```python
from build123d import *

# Parameters (mm, degrees)
F0_W     = 48
F0_H     = 1.6
F1_DEPTH = 48
F2_R     = 1.75
F2_R_2   = 1.8
F2_R_3   = 0.5
F3_DEPTH = 1.601
F4_W     = 48
F4_H     = 48
F4_R     = 1.75
F4_W_2   = 20
F4_H_2   = 9
F5_DEPTH = 5


with BuildPart() as f1:
    # F0 (on Right) → F1 (new body)
    with BuildSketch(Plane.YZ):
        Rectangle(F0_W, F0_H)
    extrude(amount=-F1_DEPTH)

    # F2 (on face) → F3 (cut, through all)
    with BuildSketch(Plane.XY.offset(0.8)):
        with Locations((-43, -19)):
            Circle(F2_R)
        with Locations((-43, 19)):
            Circle(F2_R)
        with Locations((-43.38, -9)):
            Circle(F2_R_2)
        with Locations((-4.62, -9)):
            Circle(F2_R_2)
        with Locations((-5, 19)):
            Circle(F2_R)
        with Locations((-5, -19)):
            Circle(F2_R)
        with Locations((-24, -9)):
            Circle(F2_R_3)
    extrude(amount=-F3_DEPTH, mode=Mode.SUBTRACT)


with BuildPart() as f5:
    # F4 (on Top) → F5 (new body)
    with BuildSketch(Plane.XY):
        Rectangle(F4_W, F4_H)
        with Locations((-19, -19)):
            Circle(F4_R, mode=Mode.SUBTRACT)
        with Locations((19, -19)):
            Circle(F4_R, mode=Mode.SUBTRACT)
        with Locations((-19, 19)):
            Circle(F4_R, mode=Mode.SUBTRACT)
        with Locations((0, 14.5)):
            Rectangle(F4_W_2, F4_H_2, mode=Mode.SUBTRACT)
        with Locations((19, 19)):
            Circle(F4_R, mode=Mode.SUBTRACT)
    extrude(amount=F5_DEPTH)


solid = f1.part
```
Check sheet for the modelled part. Datum: model origin and axes. Units: mm. Round coordinates to 2 decimals unless told otherwise and drop trailing zeros. Order: outer loops, then holes, each group sorted by start corner. A loop starts at its lowest first (then second) coordinate and runs counter-clockwise, first axis right, second up. Notation, with made-up numbers: M -10.5,-13 L 7.5,-13 A14 ccw 7.5,-4 Z; hole C -29,80 d2. An arc over 180 degrees is marked long. Answer in a Markdown table with one row per item.
(1) Draft check along Y on faces 1 (the cylindrical face through (-41.331, 19.526, 0.011)), 2 (the flat face through (-24, -24, 0)), 3 (the flat face through (-24, 0, 0.8)). Enter one of: +Y half, -Y half, draft (parallel to the pull), parting line (faces both ways), or undercut.
Findings:
| item | result |
|---|---|
| face 1 | undercut |
| face 2 | -Y half |
| face 3 | draft |
(2) Section check B-B on y = 18. Record the boundary of the cut face in (x, z).
Findings:
| item | result |
|---|---|
| outline | M -48,-0.8 L -44.44,-0.8 L -44.44,0.8 L -48,0.8 Z; M -41.56,-0.8 L -6.44,-0.8 L -6.44,0.8 L -41.56,0.8 Z; M -3.56,-0.8 L 0,-0.8 L 0,0.8 L -3.56,0.8 Z |
(3) Section check C-C on x = -4. Record the boundary of the cut face in (y, z), plus the area to 3 significant figures.
Findings:
| item | result |
|---|---|
| outline | M -24,-0.8 L -20.44,-0.8 L -20.44,0.8 L -24,0.8 Z; M -17.56,-0.8 L -10.69,-0.8 L -10.69,0.8 L -17.56,0.8 Z; M -7.31,-0.8 L 17.56,-0.8 L 17.56,0.8 L -7.31,0.8 Z; M 20.44,-0.8 L 24,-0.8 L 24,0.8 L 20.44,0.8 Z |
| area | 62.2 mm^2 |
(4) Section check A-A on z = 0. Record the boundary of the cut face in (x, y), plus the area to 3 significant figures.
Findings:
| item | result |
|---|---|
| outline | M -48,-24 L 0,-24 L 0,24 L -48,24 Z; hole C -43.38,-9 d3.6; hole C -43,-19 d3.5; hole C -43,19 d3.5; hole C -24,-9 d1; hole C -5,-19 d3.5; hole C -5,19 d3.5; hole C -4.62,-9 d3.6 |
| area | 2,240 mm^2 |
(5) Material ranges on line 1 along Y through (x, z) = (-4.5, -0.65); line 2 along Y through (x, z) = (-6, -0.4); line 3 along X through (y, z) = (19.5, -0.35), recorded low to high. Write a range as from..to.
Findings:
| item | result |
|---|---|
| line 1 | y = -24..-20.68, -17.32..-10.8, -7.2..17.32, 20.68..24 |
| line 2 | y = -24..-20.44, -17.56..-10.16, -7.84..17.56, 20.44..24 |
| line 3 | x = -48..-44.68, -41.32..-6.68, -3.32..0 |
(6) Section check D-D on x = -43.38. Record the boundary of the cut face in (y, z), plus the area to 3 significant figures.
Findings:
| item | result |
|---|---|
| outline | M -24,-0.8 L -20.71,-0.8 L -20.71,0.8 L -24,0.8 Z; M -17.29,-0.8 L -10.8,-0.8 L -10.8,0.8 L -17.29,0.8 Z; M -7.2,-0.8 L 17.29,-0.8 L 17.29,0.8 L -7.2,0.8 Z; M 20.71,-0.8 L 24,-0.8 L 24,0.8 L 20.71,0.8 Z |
| area | 60.1 mm^2 |
(7) Gauge pin test, flat ends, axial feed: pin 1 (3 mm diameter, centred on x = -43, y = 19, fed in from -Z); pin 2 (4 mm diameter, centred on x = -5, y = -19, fed in from +Z). Record the tip position at first contact, or that the pin passes through.
Findings:
| item | result |
|---|---|
| pin 1 | passes through |
| pin 2 | stops at z = 0.8 |
